The figure shows three views and two pictorial views of one solid part (mm, origin at its lowest corner). Answer the questions. A direction names the side the tool comes from. Round coordinates to 2 decimals unless told otherwise and drop trailing zeros. Loops run counter-clockwise (first coordinate to the right, second up) from the corner with the lowest first, then second, coordinate; pieces in that order, holes last. Notation, with made-up numbers: (30, 16) - (38, 16) arc R23 ccw to (38, 33) - close; hole circle Ø10 at (74.25, 6). An arc over 180 degrees is marked (long way). Use one line per item in the form item = value. Start each with the question number.
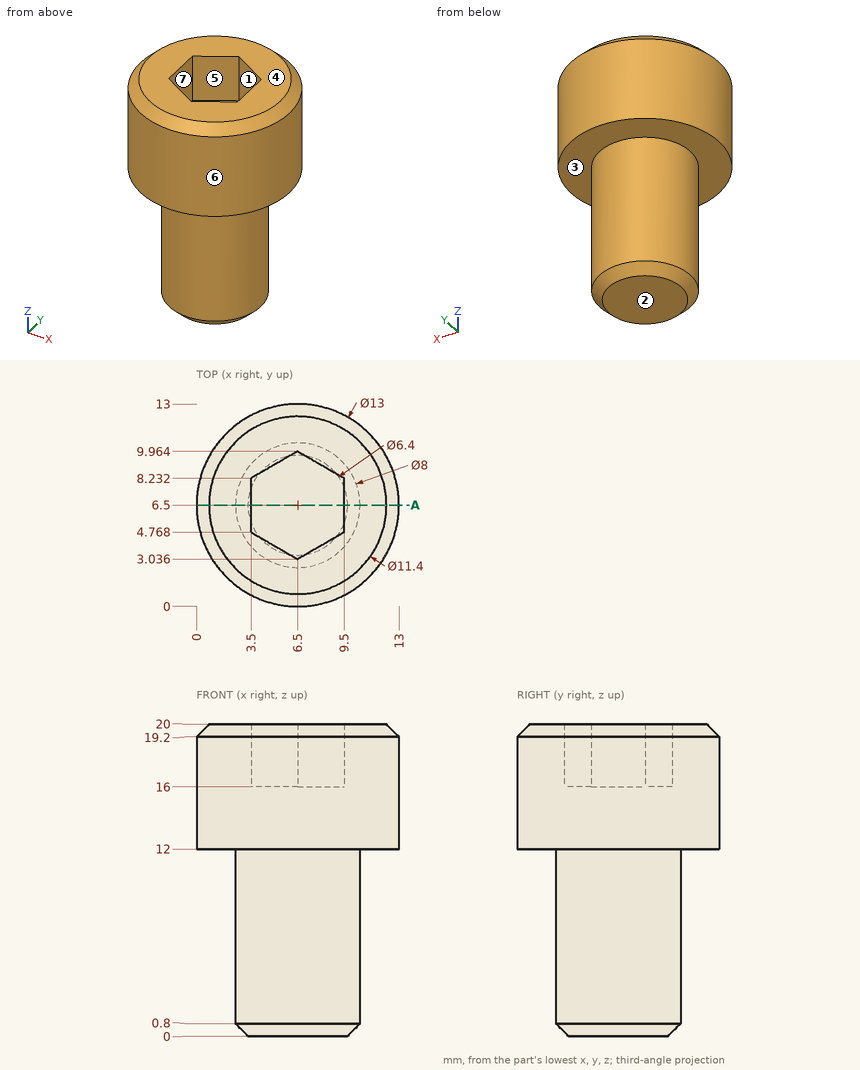
1) Straight lines are drawn through the part: line 1 (Z direction, x = 1, y = 5.25); line 2 (X direction, y = 8.5, z = 7); line 3 (Y direction, x = 7.5, z = 19). For each, find the intervals that lie inside material, in ascending order. Write a range as from..to.
2) For the marked faces 1, 2 and 3, determine the directions among +Z, -Z, +X, -X, +Y, -Y from which every point of the face is accessible in a straight line to the end or side of a thin tool.
3) Determine the mould class of the marked faces 4, 5, 6 and 7 for opening direction X: +X half, -X half, draft (parallel to the pull), parting line (faces both ways), or undercut.
4) A cutting plane is placed at A-A on y = 6.5. Write down the section's boundary in (x, z).
5) Flat-ended cylindrical pins translate along their axes: pin 1 (6.5 mm diameter, centred on x = 6.5, y = 8, fed in from +Z); pin 2 (6 mm diameter, centred on x = 3, z = 3.5, fed in from -Y); pin 3 (2 mm diameter, centred on x = 9, z = 13.5, fed in from +Y); pin 4 (6 mm diameter, centred on y = 4, z = 7.5, fed in from +X). Find the tip coordinate at first contact, or state that the pin passes through.
Checks:
q1.line_1 = 12..20
q1.line_2 = 3.04..9.96
q1.line_3 = 0.08..3.61, 9.39..12.92
q2.face_1 = +Z
q2.face_2 = -Z, +X, -X, +Y, -Y
q2.face_3 = -Z
q3.face_4 = draft
q3.face_5 = undercut
q3.face_6 = parting line
q3.face_7 = undercut
q4.outline = (0, 12) - (2.5, 12) - (2.5, 0.8) - (3.3, 0) - (9.7, 0) - (10.5, 0.8) - (10.5, 12) - (13, 12) - (13, 19.2) - (12.2, 20) - (9.5, 20) - (9.5, 16) - (3.5, 16) - (3.5, 20) - (0.8, 20) - (0, 19.2) - close
q5.pin_1 = 20
q5.pin_2 = 2.53
q5.pin_3 = 12.82
q5.pin_4 = 10.5
